from build123d import *

# Parameters (mm, degrees)
BOSS_EXTRU_1_DEPTH      = 12
COQUE5_T                = -2
ENL_V_MAT_EXTRU_1_DEPTH = 2
ESQUISSE7_R             = 1.5
ENL_V_MAT_EXTRU_2_DEPTH = 65.93843238
ESQUISSE8_R             = 1.5
ENL_V_MAT_EXTRU_3_DEPTH = 65.938432536


with BuildPart() as part:
    # Esquisse1 → Boss.-Extru.1 (new body)
    with BuildSketch(Plane.XY):
        with BuildLine():
            Line((5, 0), (47, 0))
            ThreePointArc((47, 0), (50.535533906, 1.464466094), (52, 5))
            Line((52, 5), (52, 32))
            ThreePointArc((52, 32), (50.535533906, 35.535533906), (47, 37))
            Line((47, 37), (5, 37))
            ThreePointArc((5, 37), (1.464466094, 35.535533906), (0, 32))
            Line((0, 32), (0, 5))
            ThreePointArc((0, 5), (1.464466094, 1.464466094), (5, 0))
        make_face()
    extrude(amount=BOSS_EXTRU_1_DEPTH)

    # Coque5
    coque5_openings = [part.faces().sort_by_distance(p)[0] for p in [
        (26, 18.5, 12),
    ]]
    offset(amount=COQUE5_T, openings=coque5_openings, kind=Kind.INTERSECTION)

    # Esquisse3 → Enlèv. mat.-Extru.1 (cut)
    with BuildSketch(Plane.XY.offset(12)):
        with BuildLine():
            ThreePointArc((51, 32), (49.828427125, 34.828427125), (47, 36))
            Line((47, 36), (5, 36))
            ThreePointArc((5, 36), (2.171572875, 34.828427125), (1, 32))
            Line((1, 32), (1, 5))
            ThreePointArc((1, 5), (2.171572875, 2.171572875), (5, 1))
            Line((5, 1), (47, 1))
            ThreePointArc((47, 1), (49.828427125, 2.171572875), (51, 5))
            Line((51, 5), (51, 32))
        make_face()
    extrude(amount=-ENL_V_MAT_EXTRU_1_DEPTH, mode=Mode.SUBTRACT)

    # Esquisse7 → Enlèv. mat.-Extru.2 (cut, through all)
    with BuildSketch(Plane(origin=(52, 0, 0), x_dir=(0, 0, -1), z_dir=(1, 0, 0))):
        with Locations((-6, 36.365)):
            Circle(ESQUISSE7_R)
    extrude(amount=-ENL_V_MAT_EXTRU_2_DEPTH, mode=Mode.SUBTRACT)

    # Esquisse8 → Enlèv. mat.-Extru.3 (cut, through all)
    with BuildSketch(Plane(origin=(52, 0, 0), x_dir=(0, 0, -1), z_dir=(1, 0, 0))):
        with Locations((-6, 0.635)):
            Circle(ESQUISSE8_R)
    extrude(amount=-ENL_V_MAT_EXTRU_3_DEPTH, mode=Mode.SUBTRACT)


solid = part.part
Work out the finished part from the listing and answer in its coordinate system (mm). A direction names the side the tool comes from. Coordinates: 2 decimals unless noted, no trailing zeros. Write each loop counter-clockwise with the first axis right and the second up, starting at its lowest first coordinate (ties: lowest second). Pieces come first, ordered by that corner, then holes.
1. Consider line 1 along X through (y, z) = (18.5, 3.75); line 2 along Y through (x, z) = (5, 3.75); line 3 along Z through (x, y) = (12, 29). Determine where each line is inside the solid, lowest interval first.
Results list:
line 1: x = 0 to 2, 50 to 52
line 2: y = 0 to 2, 35 to 37
line 3: z = 0 to 2
2. A flat-ended cylindrical pin translates along its axis: pin 1 (17.5 mm diameter, centred on x = 21.5, y = 25.5, fed in from +Z). Find the tip coordinate at first contact, or state that the pin passes through.
Results list:
pin 1: stops at z = 2
3. For a pull along X with two mould halves and no side action, classify faces 1 (the cylindrical face through (51.554, 34.063, 5.916)), 2 (the flat face through (26, 19, 2)), 3 (the cylindrical face through (26.351, 35.457, 7.194)) as +X half, -X half, draft (parallel to the pull), parting line (faces both ways), or undercut.
Results list:
face 1: +X half
face 2: undercut
face 3: draft
4. The part is cut by section C-C, the plane x = 27. Write down the section's boundary in (y, z) (3 decimals).
Results list:
outline: (0, 0) - (37, 0) - (37, 4.641) arc R1.5 cw to (35, 5.378) - (35, 2) - (2, 2) - (2, 5.378) arc R1.5 cw to (0, 4.641) - close; (0, 7.359) arc R1.5 cw to (2, 6.622) - (2, 10) - (1, 10) - (1, 12) - (0, 12) - close; (35, 6.622) arc R1.5 cw to (37, 7.359) - (37, 12) - (36, 12) - (36, 10) - (35, 10) - close
5. The part is cut by section A-A, the plane y = 13.5. Write down the section's boundary in (x, z), and give its area (3 significant figures).
Results list:
outline: (0, 0) - (52, 0) - (52, 12) - (51, 12) - (51, 10) - (50, 10) - (50, 2) - (2, 2) - (2, 10) - (1, 10) - (1, 12) - (0, 12) - close
area: 140 mm2
6. The part is cut by section D-D, the plane z = 6. Write down the section's boundary in (x, y) (3 decimals), and give its area (3 significant figures).
Results list:
outline: (0, 5) arc R5 ccw to (0.902, 2.135) - (4.11, 2.135) arc R3 cw to (2, 5) - (2, 32) arc R3 cw to (4.11, 34.865) - (0.902, 34.865) arc R5 ccw to (0, 32) - close; (47.89, 2.135) - (51.098, 2.135) arc R5 ccw to (52, 5) - (52, 32) arc R5 ccw to (51.098, 34.865) - (47.89, 34.865) arc R3 cw to (50, 32) - (50, 5) arc R3 cw to start
area: 134 mm2
7. For faces 4 (the cylindrical face through (49.14, 34.1, 5.94)), 5 (the flat face through (26, 37, 2)), determine the directions among +Z, -Z, +X, -X, +Y, -Y from which every point of the face is accessible in a straight line to the end or side of a thin tool.
Results list:
face 4: +Z
face 5: +Z, -Z, +X, -X, +Y
8. The part is cut by section B-B, the plane z = 9.25. Write down the section's boundary in (x, y), and give its area (3 significant figures).
Results list:
outline: (0, 5) arc R5 ccw to (5, 0) - (47, 0) arc R5 ccw to (52, 5) - (52, 32) arc R5 ccw to (47, 37) - (5, 37) arc R5 ccw to (0, 32) - close; hole (2, 5) arc R3 ccw to (5, 2) - (47, 2) arc R3 ccw to (50, 5) - (50, 32) arc R3 ccw to (47, 35) - (5, 35) arc R3 ccw to (2, 32) - close
area: 326 mm2
